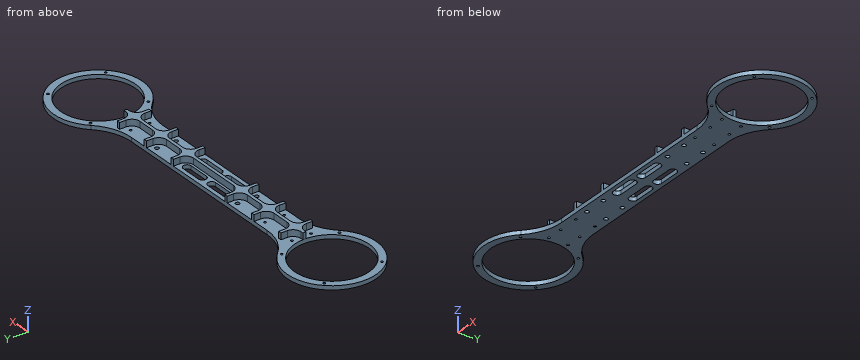
```python
from build123d import *

# Parameters (mm, degrees)
SKETCH_1_R           = 47
EXTRUDE_1_DEPTH      = 5
FILLET_1_R           = 60
SKETCH_31_R          = 1.5
CUT_EXTRUDE_14_DEPTH = 5
SKETCH_32_W          = 306
SKETCH_32_H          = 4
EXTRUDE_2_DEPTH      = 8
CUT_EXTRUDE_17_DEPTH = 8
SKETCH_35_R          = 2.5
CUT_EXTRUDE_18_DEPTH = 10
EXTRUDE_3_DEPTH      = 5
SKETCH_37_R          = 1.5
CUT_EXTRUDE_19_DEPTH = 10
SKETCH_38_W          = 4
SKETCH_38_H          = 40
EXTRUDE_4_DEPTH      = 8
FILLET_2_R           = 10
SKETCH_41_R          = 1.5
SKETCH_41_R_2        = 2.5
CUT_EXTRUDE_20_DEPTH = 10


with BuildPart() as part:
    # 草图1 → 凸台-拉伸1 (new body)
    with BuildSketch(Plane.XY):
        with BuildLine():
            Line((347.693212678, 20), (52.306787322, 20))
            ThreePointArc((52.306787322, 20), (-56, 0), (52.306787322, -20))
            Line((52.306787322, -20), (347.693212678, -20))
            ThreePointArc((347.693212678, -20), (456, 0), (347.693212678, 20))
        make_face()
        Circle(SKETCH_1_R, mode=Mode.SUBTRACT)
        with Locations((400, 0)):
            Circle(SKETCH_1_R, mode=Mode.SUBTRACT)
    extrude(amount=EXTRUDE_1_DEPTH)

    # 圆角1
    fillet_1_edges = [part.edges().sort_by_distance(p)[0] for p in [
        (347.693212678, -20, 2.5),
        (52.306787322, -20, 2.5),
        (52.306787322, 20, 2.5),
        (347.693212678, 20, 2.5),
    ]]
    fillet(fillet_1_edges, radius=FILLET_1_R)

    # 草图31 → 切除-拉伸14 (cut)
    with BuildSketch(Plane.XY.offset(5)):
        with Locations((36.415999231, 36.415999231)):
            Circle(SKETCH_31_R)
        with Locations((36.415999231, -36.415999231)):
            Circle(SKETCH_31_R)
        with Locations((-36.415999231, -36.415999231)):
            Circle(SKETCH_31_R)
        with Locations((-36.415999231, 36.415999231)):
            Circle(SKETCH_31_R)
        with Locations(Location((436.415999231, 36.415999231, 0), (0, 0, 180))):
            Circle(SKETCH_31_R)
        with Locations(Location((436.415999231, -36.415999231, 0), (0, 0, 180))):
            Circle(SKETCH_31_R)
        with Locations(Location((363.584000769, -36.415999231, 0), (0, 0, 180))):
            Circle(SKETCH_31_R)
        with Locations(Location((363.584000769, 36.415999231, 0), (0, 0, 180))):
            Circle(SKETCH_31_R)
    extrude(amount=-CUT_EXTRUDE_14_DEPTH, mode=Mode.SUBTRACT)

    # 草图32 → 凸台-拉伸2 (add)
    with BuildSketch(Plane.XY.offset(5)):
        with Locations((200, 0)):
            Rectangle(SKETCH_32_W, SKETCH_32_H)
    extrude(amount=EXTRUDE_2_DEPTH)

    # 草图34 → 切除-拉伸17 (cut)
    with BuildSketch(Plane.XY.offset(5)):
        with BuildLine():
            Line((164, 5), (192, 5))
            ThreePointArc((192, 5), (197, 10), (192, 15))
            Line((192, 15), (164, 15))
            ThreePointArc((164, 15), (159, 10), (164, 5))
        make_face()
        with BuildLine():
            Line((164, -15), (192, -15))
            ThreePointArc((192, -15), (197, -10), (192, -5))
            Line((192, -5), (164, -5))
            ThreePointArc((164, -5), (159, -10), (164, -15))
        make_face()
        with BuildLine():
            Line((208, 15), (236, 15))
            ThreePointArc((236, 15), (241, 10), (236, 5))
            Line((236, 5), (208, 5))
            ThreePointArc((208, 5), (203, 10), (208, 15))
        make_face()
        with BuildLine():
            Line((208, -5), (236, -5))
            ThreePointArc((236, -5), (241, -10), (236, -15))
            Line((236, -15), (208, -15))
            ThreePointArc((208, -15), (203, -10), (208, -5))
        make_face()
    extrude(amount=-CUT_EXTRUDE_17_DEPTH, mode=Mode.SUBTRACT)

    # 草图35 → 切除-拉伸18 (cut)
    with BuildSketch(Plane.XY.offset(5)):
        with Locations((145, 12)):
            Circle(SKETCH_35_R)
        with Locations((145, -12)):
            Circle(SKETCH_35_R)
        with Locations((255, 12)):
            Circle(SKETCH_35_R)
        with Locations((255, -12)):
            Circle(SKETCH_35_R)
    extrude(amount=-CUT_EXTRUDE_18_DEPTH, mode=Mode.SUBTRACT)

    # 草图36 → 凸台-拉伸3 (add)
    with BuildSketch(Plane.XY.offset(5)):
        with BuildLine():
            Line((164, 15), (166, 15))
            ThreePointArc((166, 15), (161, 10), (166, 5))
            Line((166, 5), (164, 5))
            ThreePointArc((164, 5), (159, 10), (164, 15))
        make_face()
        with BuildLine():
            Line((164, -5), (166, -5))
            ThreePointArc((166, -5), (161, -10), (166, -15))
            Line((166, -15), (164, -15))
            ThreePointArc((164, -15), (159, -10), (164, -5))
        make_face()
        with BuildLine():
            Line((234, 15), (236, 15))
            ThreePointArc((236, 15), (241, 10), (236, 5))
            Line((236, 5), (234, 5))
            ThreePointArc((234, 5), (239, 10), (234, 15))
        make_face()
        with BuildLine():
            Line((234, -5), (236, -5))
            ThreePointArc((236, -5), (241, -10), (236, -15))
            Line((236, -15), (234, -15))
            ThreePointArc((234, -15), (239, -10), (234, -5))
        make_face()
    extrude(amount=-EXTRUDE_3_DEPTH)

    # 草图37 → 切除-拉伸19 (cut)
    with BuildSketch(Plane.XY.offset(5)):
        with Locations((72.001998556, -12.000000249)):
            Circle(SKETCH_37_R)
        with Locations((72.001998556, 11.999999751)):
            Circle(SKETCH_37_R)
        with Locations((52.000000094, -12.000000249)):
            Circle(SKETCH_37_R)
        with Locations((52.000000094, 11.999999751)):
            Circle(SKETCH_37_R)
        with Locations((347.999999906, 11.999999751)):
            Circle(SKETCH_37_R)
        with Locations((347.999999906, -12.000000249)):
            Circle(SKETCH_37_R)
        with Locations((327.998001444, 11.999999751)):
            Circle(SKETCH_37_R)
        with Locations((327.998001444, -12.000000249)):
            Circle(SKETCH_37_R)
    extrude(amount=-CUT_EXTRUDE_19_DEPTH, mode=Mode.SUBTRACT)

    # 草图38 → 凸台-拉伸4 (add)
    with BuildSketch(Plane.XY.offset(5)):
        with Locations((62.000999325, 0)):
            Rectangle(SKETCH_38_W, SKETCH_38_H)
        with Locations((108.000999325, 0)):
            Rectangle(SKETCH_38_W, SKETCH_38_H)
        with Locations((154.000999325, 0)):
            Rectangle(SKETCH_38_W, SKETCH_38_H)
        with Locations((245.999000675, 0)):
            Rectangle(SKETCH_38_W, SKETCH_38_H)
        with Locations((291.999000675, 0)):
            Rectangle(SKETCH_38_W, SKETCH_38_H)
        with Locations((337.999000675, 0)):
            Rectangle(SKETCH_38_W, SKETCH_38_H)
    extrude(amount=EXTRUDE_4_DEPTH)

    # 圆角2
    fillet_2_edges = [part.edges().sort_by_distance(p)[0] for p in [
        (64.000999325, 2, 9),
        (64.000999325, -2, 9),
        (60.000999325, 2, 9),
        (60.000999325, -2, 9),
        (110.000999325, 2, 9),
        (110.000999325, -2, 9),
        (106.000999325, 2, 9),
        (106.000999325, -2, 9),
        (156.000999325, 2, 9),
        (156.000999325, -2, 9),
        (152.000999325, 2, 9),
        (152.000999325, -2, 9),
        (247.999000675, 2, 9),
        (247.999000675, -2, 9),
        (243.999000675, 2, 9),
        (243.999000675, -2, 9),
        (293.999000675, 2, 9),
        (293.999000675, -2, 9),
        (289.999000675, 2, 9),
        (289.999000675, -2, 9),
        (339.999000675, 2, 9),
        (339.999000675, -2, 9),
        (335.999000675, 2, 9),
        (335.999000675, -2, 9),
    ]]
    fillet(fillet_2_edges, radius=FILLET_2_R)

    # 草图41 → 切除-拉伸20 (cut)
    with BuildSketch(Plane.XY.offset(5)):
        with Locations((327.998001444, -12.000000249)):
            Circle(SKETCH_41_R)
        with Locations((327.998001444, 11.999999751)):
            Circle(SKETCH_41_R)
        with Locations((255, -12)):
            Circle(SKETCH_41_R_2)
        with Locations((255, 12)):
            Circle(SKETCH_41_R_2)
        with Locations((145, -12)):
            Circle(SKETCH_41_R_2)
        with Locations((145, 12)):
            Circle(SKETCH_41_R_2)
        with Locations((72.001998556, -12.000000249)):
            Circle(SKETCH_41_R)
        with Locations((72.001998556, 11.999999751)):
            Circle(SKETCH_41_R)
        with Locations((98.000000094, -12.000000249)):
            Circle(SKETCH_41_R)
        with Locations((98.000000094, 11.999999751)):
            Circle(SKETCH_41_R)
        with Locations((117.001998651, -12)):
            Circle(SKETCH_41_R_2)
        with Locations((117.001998651, 12)):
            Circle(SKETCH_41_R_2)
        with Locations((282.998001349, -12)):
            Circle(SKETCH_41_R_2)
        with Locations((282.998001349, 12)):
            Circle(SKETCH_41_R_2)
        with Locations((301.999999906, -12.000000249)):
            Circle(SKETCH_41_R)
        with Locations((301.999999906, 11.999999751)):
            Circle(SKETCH_41_R)
    extrude(amount=-CUT_EXTRUDE_20_DEPTH, mode=Mode.SUBTRACT)


solid = part.part
```
Model file for the job. Use its own axes, mm. Coordinates: 2 decimals unless noted, no trailing zeros. Loops run counter-clockwise (first coordinate to the right, second up) from the corner with the lowest first, then second, coordinate; pieces in that order, holes last. Notation, with made-up numbers: (14.25, 79) - (27.25, 79) arc R16 cw to (27.25, 98) - close; hole circle Ø4 at (4, 66.5). An arc over 180 degrees is marked (long way). Write item = value, one per line. Start each with the question number.
Item 1: Drop flat-ended pins along their axis: pin 1 Ø3 at (x, z) = (224, 7) entering from +Y; pin 2 Ø2.5 at (y, z) = (15.5, 7) entering from -X; pin 3 Ø5 at (y, z) = (10.5, 3) entering from -X. Give the stop position or say it passes through.
Item 2: Saw through at C-C, the plane x = 409. List the corners of the cut face in (y, z), then the cut area to 3 significant figures.
Item 3: Saw through at D-D, the plane z = 3. State how many separate pieces and enclosed holes the cut face has, then the cut area to 3 significant figures.
Item 4: Saw through at A-A, the plane x = 0. List the corners of the cut face in (y, z).
Item 5: Wall check: probe 1 along Y at (x, z) = (145, 3.9); probe 2 along X at (y, z) = (-13, 12.5); probe 3 along X at (y, z) = (43, 1.5). Give the ranges that are in metal, low to high. Write a range as [from, to].
Item 6: Saw through at B-B, the plane x = 268. List the corners of the cut face in (y, z).
Answers:
q1.pin_1 = 2
q1.pin_2 = 60
q1.pin_3 = -55.43
q2.outline = (-55.27, 0) - (-46.13, 0) - (-46.13, 5) - (-55.27, 5) - close; (46.13, 0) - (55.27, 0) - (55.27, 5) - (46.13, 5) - close
q2.area = 91.4 mm2
q3.separate_pieces = 1
q3.enclosed_holes = 34
q3.area = 16,300 mm2
q4.outline = (-56, 0) - (-47, 0) - (-47, 5) - (-56, 5) - close; (47, 0) - (56, 0) - (56, 5) - (47, 5) - close
q5.probe_1 = [-20, -14.5], [-9.5, 9.5], [14.5, 20]
q5.probe_2 = [60, 64], [106, 110], [152, 156], [244, 248], [290, 294], [336, 340]
q5.probe_3 = [-35.87, -18.97], [18.97, 35.87], [364.13, 381.03], [418.97, 435.87]
q6.outline = (-20, 0) - (20, 0) - (20, 5) - (2, 5) - (2, 13) - (-2, 13) - (-2, 5) - (-20, 5) - close
